Source: CAD feature listing. Evaluate the final solid. Frame: model axes, mm. Face numbers are marked on the shaded views. Round coordinates to 2 decimals unless told otherwise and drop trailing zeros. Loops run counter-clockwise (first coordinate to the right, second up) from the corner with the lowest first, then second, coordinate; pieces in that order, holes last. Notation, with made-up numbers: (52.25, -19) -> (61.25, -19) arc R20 ccw to (61.25, 20) -> close; hole circle Ø8 at (11.5, 62.5). An arc over 180 degrees is marked (long way). Put each result on its own line as item: value. Start each with the question number.
1. Contact query for flat-ended pins moving along their axis: pin 1 (4 mm diameter, centred on x = 134, y = 53, fed in from +Z); pin 2 (2 mm diameter, centred on x = 116, y = 70, fed in from +Z); pin 3 (3 mm diameter, centred on y = 33.5, z = 84.5, fed in from -X); pin 4 (5 mm diameter, centred on x = 35.5, z = 10, fed in from +Y). Output: stop coordinate, or through.
2. Cut plane A-A (x = 23.5). Return the cut outline in (y, z) (3 decimals), then the cut area to 3 significant figures.
3. Draft query along Y for the marked faces 1 and 2. Return one class per face: pulls with the +Y half, pulls with the -Y half, needs draft (parallel to the pull), parting line crosses it, or undercut.
4. Material intervals for L1, parallel to Z at x = 33, y = 84; L2, parallel to Y at x = 134, z = 7; L3, parallel to Z at x = 152, y = 75, sorted ascending.
5. Cut plane C-C (z = 62). Return the cut outline in (x, y).
6. Cut plane B-B (y = 42). Return the cut outline in (x, z).
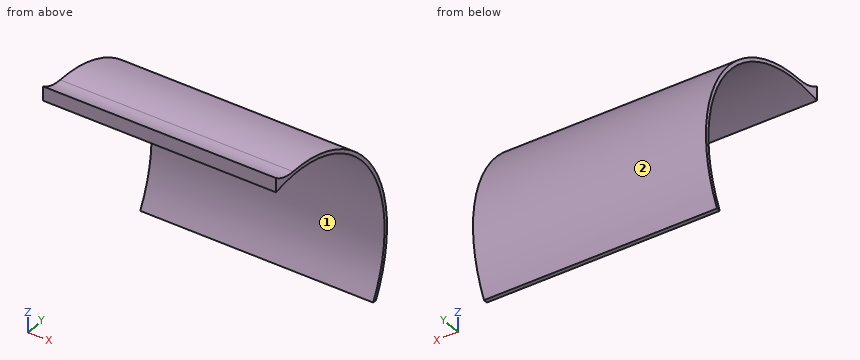
```python
from build123d import *

# Parameters (mm, degrees)
SALIENTE_EXTRUIR1_DEPTH = 160
SALIENTE_EXTRUIR3_START = -160
SALIENTE_EXTRUIR3_DEPTH = 160


with BuildPart() as part:
    # Croquis1 → Saliente-Extruir1 (new body)
    with BuildSketch(Plane(origin=(0, 0, 0), x_dir=(0, 0, -1), z_dir=(1, 0, 0))):
        with BuildLine():
            ThreePointArc((45, 84.539297963), (-56.606836573, 77.249977043), (-94.168674728, -17.44))
            Line((-94.168674728, -17.44), (-91.624992769, -17.44))
            ThreePointArc((-91.624992769, -17.44), (-54.7766031, 75.490507038), (45, 81.696345696))
            Line((45, 81.696345696), (45, 84.539297963))
        make_face()
    extrude(amount=SALIENTE_EXTRUIR1_DEPTH)

    # Croquis2 → Saliente-Extruir3 (add)
    with BuildSketch(Plane(origin=(160, 0, 0), x_dir=(0, 0, -1), z_dir=(1, 0, 0)).offset(SALIENTE_EXTRUIR3_START)):
        with BuildLine():
            Line((-94.168674728, -17.44), (-101.624992769, -17.44))
            ThreePointArc((-101.624992769, -17.44), (-97.2728202, -9.198295227), (-95.77, 0))
            ThreePointArc((-95.77, 0), (-95.368828447, -8.756680916), (-94.168674728, -17.44))
        make_face()
    extrude(amount=SALIENTE_EXTRUIR3_DEPTH)


solid = part.part
```
Solution:
1. pin 1: stops at z = 81.06
1. pin 2: stops at z = 66.41
1. pin 3: passes through
1. pin 4: stops at y = 95.48
2. outline: (-17.44, 91.625) arc R93.27 cw to (81.696, -45) -> (84.539, -45) arc R95.77 ccw to (0, 95.77) arc R28.901 cw to (-17.44, 101.625) -> close
2. area: 574 mm^2
3. face 1: undercut
3. face 2: pulls with the +Y half
4. L1: z = -45 to -40.54, 40.54 to 46
4. L2: y = 93.01 to 95.51
4. L3: z = 55.45 to 59.56
5. outline: (0, 69.68) -> (160, 69.68) -> (160, 72.99) -> (0, 72.99) -> close
6. outline: (0, 83.28) -> (160, 83.28) -> (160, 86.07) -> (0, 86.07) -> close
